Here's how the part is built. I have some questions about the finished solid (model axes, mm). Face numbers are marked on the shaded views. Give positions to 0.01 mm unless a question says otherwise; leave off trailing zeros. Loops run counter-clockwise (first coordinate to the right, second up) from the corner with the lowest first, then second, coordinate; pieces in that order, holes last.
Q1. I'm going to push flat-ended pins straight in: P1, Ø2.5, axis at x = -19.5, z = 2, coming from the -Y side; P2, Ø2.5, axis at x = -29, z = 0, coming from the +Y side; P3, Ø2.5, axis at x = 21.5, y = 47.75, coming from the -Z side. Where does each tip first touch, or does it pass through?
Q2. Thinking about a two-plate mould opening in Y: for the marked faces 1 and 2, which applies, pulls with the +Y half, pulls with the -Y half, needs draft (parallel to the pull), parting line crosses it, or undercut?
Q3. Suppose I cut it at B-B (x = -26.5). List the corners of the cut face in (y, z) for me.
Q4. Suppose I cut it at A-A (y = -6). List the corners of the cut face in (x, z) for me, and give its area (3 significant figures).
Q5. I need wall thicknesses on probe 1 along X at (y, z) = (-40.75, 2.4); probe 2 along X at (y, z) = (47.75, 2.95); probe 3 along Y at (x, z) = (35.5, -2.75). Which ranges of each line are inside material? Lowest first, please.
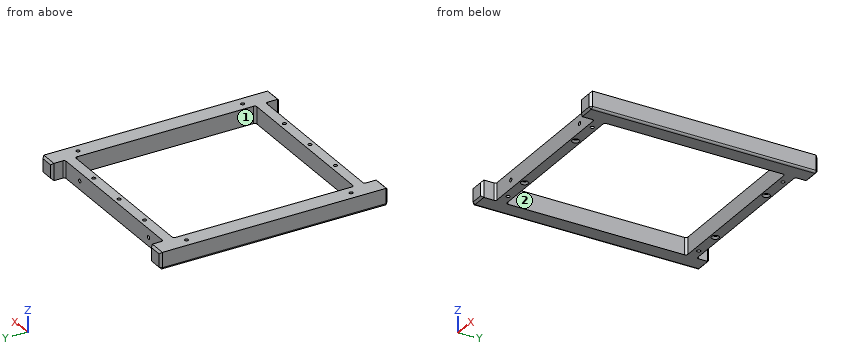
```python
from build123d import *

# Parameters (mm, degrees)
SKETCH1_W                            = 100
SKETCH1_H                            = 113.5
BOSS_EXTRUDE1_DEPTH                  = 4.25
CUT_EXTRUDE1_DEPTH                   = 77.110528181
M1_6_HOLE1_INTUNION_D                = 1.8
M1_6_HOLE1_INTUNION_DEPTH            = 5
M1_6_HOLE1_INTUNION_TIP              = 0.540774557
M1_6_HOLE2_INTUNIONPLATE_D           = 1.8
M1_6_HOLE2_INTUNIONPLATE_CSINK_D     = 3.6
M1_6_HOLE2_INTUNIONPLATE_CSINK_ANGLE = 90
M1_6_HOLE3_EXTUNIONSIDE_D            = 1.8
M1_6_HOLE3_EXTUNIONSIDE_DEPTH        = 3
M1_6_HOLE3_EXTUNIONSIDE_TIP          = 0.540774557
M1_6_HOLE4_INTUNIONTOP_D             = 1.8
M1_6_HOLE4_INTUNIONTOP_DEPTH         = 3
M1_6_HOLE4_INTUNIONTOP_TIP           = 0.540774557
M1_6_HOLE5_EXTUNIONTOP_D             = 1.8
M1_6_HOLE5_EXTUNIONTOP_DEPTH         = 2
M1_6_HOLE5_EXTUNIONTOP_TIP           = 0.540774557
M1_6_HOLE6_EXTUNIONTOP_D             = 1.8
M1_6_HOLE6_EXTUNIONTOP_DEPTH         = 3
M1_6_HOLE6_EXTUNIONTOP_TIP           = 0.540774557
FILLET1_R                            = 1
CHAMFER1_SIZE                        = 1


with BuildPart() as part:
    # Sketch1 → Boss-Extrude1 (new, symmetric)
    with BuildSketch(Plane.XY):
        Rectangle(SKETCH1_W, SKETCH1_H)
    extrude(amount=BOSS_EXTRUDE1_DEPTH, both=True)

    # Sketch4 → Cut-Extrude1 (cut, through all)
    with BuildSketch(Plane.XY.offset(4.25)):
        with BuildLine():
            Line((-40.5, -44.75), (40.5, -44.75))
            ThreePointArc((40.5, -44.75), (41.207106781, -44.457106781), (41.5, -43.75))
            Line((41.5, -43.75), (41.5, 44.25))
            ThreePointArc((41.5, 44.25), (41.207106781, 44.957106781), (40.5, 45.25))
            Line((40.5, 45.25), (-40.5, 45.25))
            ThreePointArc((-40.5, 45.25), (-41.207106781, 44.957106781), (-41.5, 44.25))
            Line((-41.5, 44.25), (-41.5, -43.75))
            ThreePointArc((-41.5, -43.75), (-41.207106781, -44.457106781), (-40.5, -44.75))
        make_face()
        with BuildLine():
            Line((-41.5, 56.75), (41.5, 56.75))
            Line((41.5, 56.75), (41.5, 51.25))
            ThreePointArc((41.5, 51.25), (41.207106781, 50.542893219), (40.5, 50.25))
            Line((40.5, 50.25), (-40.5, 50.25))
            ThreePointArc((-40.5, 50.25), (-41.207106781, 50.542893219), (-41.5, 51.25))
            Line((-41.5, 51.25), (-41.5, 56.75))
        make_face()
        with BuildLine():
            Line((-41.5, -56.75), (41.5, -56.75))
            Line((41.5, -56.75), (41.5, -50.75))
            ThreePointArc((41.5, -50.75), (41.207106781, -50.042893219), (40.5, -49.75))
            Line((40.5, -49.75), (-40.5, -49.75))
            ThreePointArc((-40.5, -49.75), (-41.207106781, -50.042893219), (-41.5, -50.75))
            Line((-41.5, -50.75), (-41.5, -56.75))
        make_face()
    extrude(amount=-CUT_EXTRUDE1_DEPTH, mode=Mode.SUBTRACT)

    # M1.6 Hole1-IntUnion
    with Locations(Plane.XY.offset(4.25)):
        with Locations((-45.75, -40.75), (45.75, -40.75), (-45.75, 41.25), (45.75, 41.25)):
            Hole(M1_6_HOLE1_INTUNION_D / 2, depth=M1_6_HOLE1_INTUNION_DEPTH)
            with Locations((0, 0, -(M1_6_HOLE1_INTUNION_DEPTH + M1_6_HOLE1_INTUNION_TIP / 2))):  # 118° drill point
                Cone(0, M1_6_HOLE1_INTUNION_D / 2, M1_6_HOLE1_INTUNION_TIP, mode=Mode.SUBTRACT)

    # M1.6 Hole2-IntUnionPlate (through all)
    with Locations(Plane(origin=(0, 0, -4.25), x_dir=(-1, 0, 0), z_dir=(0, 0, -1))):
        with Locations((-21.5, 47.75), (21.5, 47.75), (-21.5, -47.25), (21.5, -47.25)):
            CounterSinkHole(M1_6_HOLE2_INTUNIONPLATE_D / 2, M1_6_HOLE2_INTUNIONPLATE_CSINK_D / 2, counter_sink_angle=M1_6_HOLE2_INTUNIONPLATE_CSINK_ANGLE)

    # M1.6 Hole3-ExtUnionSide
    with Locations(Plane(origin=(0, 0, -4.25), x_dir=(-1, 0, 0), z_dir=(0, 0, -1))):
        with Locations((-35.5, 47.75), (35.5, 47.75), (-35.5, -47.25), (35.5, -47.25)):
            Hole(M1_6_HOLE3_EXTUNIONSIDE_D / 2, depth=M1_6_HOLE3_EXTUNIONSIDE_DEPTH)
            with Locations((0, 0, -(M1_6_HOLE3_EXTUNIONSIDE_DEPTH + M1_6_HOLE3_EXTUNIONSIDE_TIP / 2))):  # 118° drill point
                Cone(0, M1_6_HOLE3_EXTUNIONSIDE_D / 2, M1_6_HOLE3_EXTUNIONSIDE_TIP, mode=Mode.SUBTRACT)

    # M1.6 Hole4-IntUnionTop
    with Locations(Plane.XY.offset(4.25)):
        with Locations((0, 47.75), (0, -47.25)):
            Hole(M1_6_HOLE4_INTUNIONTOP_D / 2, depth=M1_6_HOLE4_INTUNIONTOP_DEPTH)
            with Locations((0, 0, -(M1_6_HOLE4_INTUNIONTOP_DEPTH + M1_6_HOLE4_INTUNIONTOP_TIP / 2))):  # 118° drill point
                Cone(0, M1_6_HOLE4_INTUNIONTOP_D / 2, M1_6_HOLE4_INTUNIONTOP_TIP, mode=Mode.SUBTRACT)

    # M1.6 Hole5-ExtUnionTop
    with Locations(Plane(origin=(0, 50.25, 0), x_dir=(1, 0, 0), z_dir=(0, 1, 0))):
        with Locations((-29, 0), (29, 0)):
            Hole(M1_6_HOLE5_EXTUNIONTOP_D / 2, depth=M1_6_HOLE5_EXTUNIONTOP_DEPTH)
            with Locations((0, 0, -(M1_6_HOLE5_EXTUNIONTOP_DEPTH + M1_6_HOLE5_EXTUNIONTOP_TIP / 2))):  # 118° drill point
                Cone(0, M1_6_HOLE5_EXTUNIONTOP_D / 2, M1_6_HOLE5_EXTUNIONTOP_TIP, mode=Mode.SUBTRACT)

    # M1.6 Hole6-ExtUnionTop
    with Locations(Plane(origin=(0, -49.75, 0), x_dir=(-1, 0, 0), z_dir=(0, -1, 0))):
        with Locations((29, 0), (-29, 0)):
            Hole(M1_6_HOLE6_EXTUNIONTOP_D / 2, depth=M1_6_HOLE6_EXTUNIONTOP_DEPTH)
            with Locations((0, 0, -(M1_6_HOLE6_EXTUNIONTOP_DEPTH + M1_6_HOLE6_EXTUNIONTOP_TIP / 2))):  # 118° drill point
                Cone(0, M1_6_HOLE6_EXTUNIONTOP_D / 2, M1_6_HOLE6_EXTUNIONTOP_TIP, mode=Mode.SUBTRACT)

    # Fillet1
    fillet1_edges = [part.edges().sort_by_distance(p)[0] for p in [
        (-50, 0, -4.25),
        (50, 0, -4.25),
    ]]
    fillet(fillet1_edges, radius=FILLET1_R)

    # Chamfer1
    chamfer1_edges = [part.edges().sort_by_distance(p)[0] for p in [
        (-45.75, -56.75, 4.25),
        (45.25, -56.75, -4.25),
        (45.75, -56.75, 4.25),
        (-45.25, -56.75, -4.25),
        (-49.707106781, -56.75, -3.957106781),
        (45.25, 56.75, -4.25),
        (-49.707106781, 56.75, -3.957106781),
        (49.707106781, 56.75, -3.957106781),
        (49.707106781, -56.75, -3.957106781),
        (41.5, -56.75, 0),
        (-41.5, -56.75, 0),
        (-45.25, 56.75, -4.25),
        (-45.75, 56.75, 4.25),
        (-41.5, 56.75, 0),
        (41.5, 56.75, 0),
        (45.75, 56.75, 4.25),
        (50, -56.75, 0.5),
        (-50, -56.75, 0.5),
        (-50, 56.75, 0.5),
        (50, 56.75, 0.5),
    ]]
    chamfer(chamfer1_edges, length=CHAMFER1_SIZE - 0.0001)  # a hair under: the kernel refuses the full size


solid = part.part
```
Solutions:
1. P1: stops at y = -49.75
1. P2: stops at y = 50.25
1. P3: stops at z = -3.7
2. face 1: undercut
2. face 2: undercut
3. outline: (-49.75, -4.25) - (-44.75, -4.25) - (-44.75, 4.25) - (-49.75, 4.25) - close; (45.25, -4.25) - (50.25, -4.25) - (50.25, 4.25) - (45.25, 4.25) - close
4. outline: (-50, -3.25) arc R1 ccw to (-49, -4.25) - (-41.5, -4.25) - (-41.5, 4.25) - (-50, 4.25) - close; (41.5, -4.25) - (49, -4.25) arc R1 ccw to (50, -3.25) - (50, 4.25) - (41.5, 4.25) - close
4. area: 144 mm2
5. probe 1: x = -50 to -46.65, -44.85 to -41.5, 41.5 to 44.85, 46.65 to 50
5. probe 2: x = -50 to -22.4, -20.6 to -0.9, 0.9 to 20.6, 22.4 to 50
5. probe 3: y = -49.75 to -48.15, -46.35 to -44.75, 45.25 to 46.85, 48.65 to 50.25
